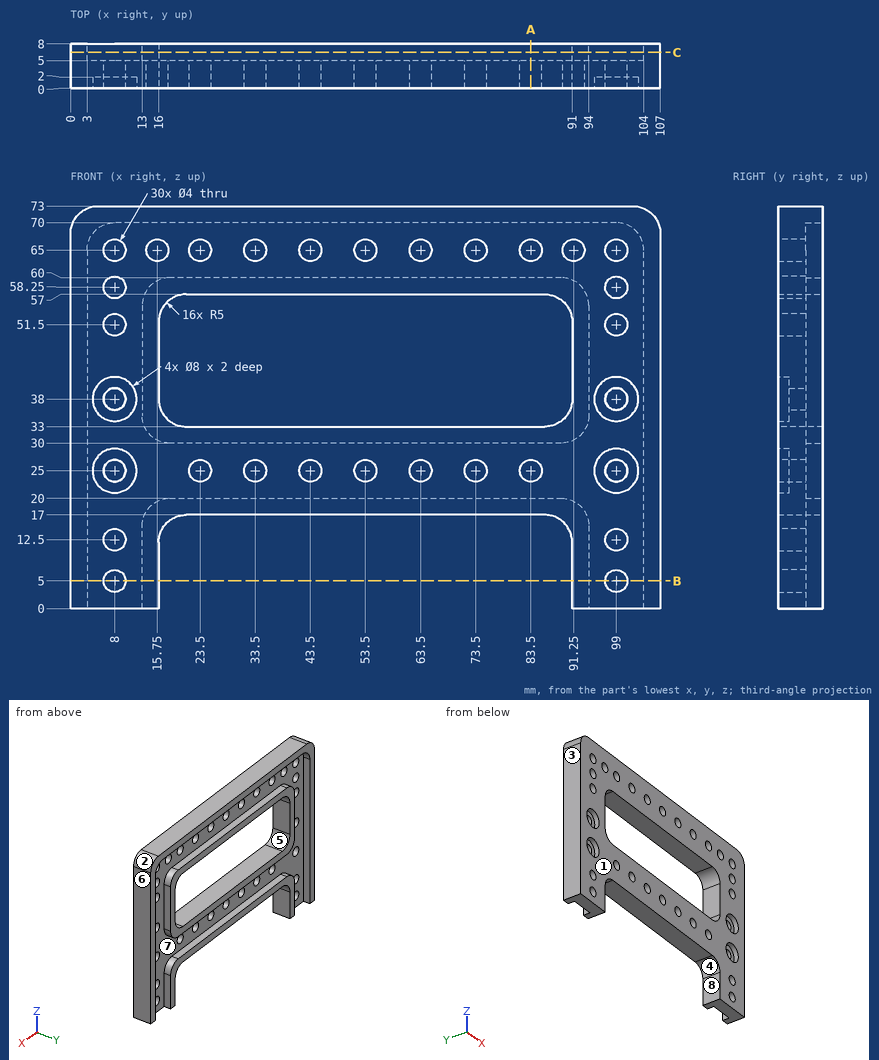
Print and shaded views of the part. All mm, measured from the part's lowest x, y and z. A direction names the side the tool comes from. Give positions to 0.01 mm unless a question says otherwise; leave off trailing zeros. Loops run counter-clockwise (first coordinate to the right, second up) from the corner with the lowest first, then second, coordinate; pieces in that order, holes last. Notation, with made-up numbers: (33, -18) - (58, -18) arc R30 ccw to (58, 17) - close; hole circle Ø9 at (40, 64). An arc over 180 degrees is marked (long way). One line per item, written item: value. Start each with the question number.
1. Slice it at A-A (x = 83.5). List the corners of the cut face in (y, z), plus the area to 3 significant figures.
2. Probe L1, parallel to X at y = 5.25, z = 52; L2, parallel to Z at x = 79, y = 7.5; L3, parallel to Z at x = 27, y = 3.5. List the from-to ranges inside material, lowest first. Write a range as from..to.
3. Which spindle directions (+Z, -Z, +X, -X, +Y, -Y) get a long thin tool onto all of the face, cutting with end or side? Do the marked faces 5, 6, 7 and 8. Say none if no direction does.
4. Pull direction X, two halves, no side cores. Call the marked faces 1, 2, 3 and 4: pulls with the +X half, pulls with the -X half, needs draft (parallel to the pull), parting line crosses it, or undercut.
5. Slice it at B-B (z = 5). List the corners of the cut face in (x, y).
6. Slice it at C-C (y = 6.5). Give the number of separate pieces and of enclosed holes in the cut face, plus the area to 3 significant figures.
7. Pin check, flat tips, straight feed: pin 1 (5 mm diameter, centred on x = 8, z = 25, fed in from -Y); pin 2 (4.5 mm diameter, centred on x = 83.5, z = 25, fed in from +Y); pin 3 (4 mm diameter, centred on x = 51.5, y = 4, fed in from -Z). Stop position of each tip, or through.
Solution:
1. outline: (0, 17) - (8, 17) - (8, 20) - (5, 20) - (5, 23) - (0, 23) - close; (0, 27) - (5, 27) - (5, 30) - (8, 30) - (8, 33) - (0, 33) - close; (0, 57) - (8, 57) - (8, 60) - (5, 60) - (5, 63) - (0, 63) - close; (0, 67) - (5, 67) - (5, 70) - (8, 70) - (8, 73) - (0, 73) - close
1. area: 156 mm^2
2. L1: x = 0..3, 13..16, 91..94, 104..107
2. L2: z = 17..20, 30..33, 57..60, 70..73
2. L3: z = 17..33, 57..73
3. face 5: +Y, -Y
3. face 6: +Z, -Z, +X, +Y, -Y
3. face 7: +Y
3. face 8: -Z, +Y, -Y
4. face 1: needs draft
4. face 2: pulls with the +X half
4. face 3: pulls with the -X half
4. face 4: undercut
5. outline: (0, 0) - (6, 0) - (6, 5) - (3, 5) - (3, 8) - (0, 8) - close; (10, 0) - (16, 0) - (16, 8) - (13, 8) - (13, 5) - (10, 5) - close; (91, 0) - (97, 0) - (97, 5) - (94, 5) - (94, 8) - (91, 8) - close; (101, 0) - (107, 0) - (107, 8) - (104, 8) - (104, 5) - (101, 5) - close
6. separate pieces: 3
6. enclosed holes: 1
6. area: 1,720 mm^2
7. pin 1: stops at y = 2
7. pin 2: stops at y = 5
7. pin 3: stops at z = 17
